from build123d import *

# Parameters (mm, degrees)
F0_W     = 62
F0_H     = 36
F1_DEPTH = 32
F2_W     = 60
F2_H     = 30
F3_DEPTH = 36.001
F5_DEPTH = 12.001
F6_W     = 16
F6_H     = 12
F7_DEPTH = 12.001
F8_R     = 8
F9_DEPTH = 12.001
F10_R    = 5


with BuildPart() as f1:
    # F0 (on Top) → F1 (new body)
    with BuildSketch(Plane.XY):
        with Locations((-13, 0)):
            Rectangle(F0_W, F0_H)
    extrude(amount=F1_DEPTH)

    # F2 (on face) → F3 (cut, through all)
    with BuildSketch(Plane.XZ.offset(18)):
        with Locations((-2, 27)):
            Rectangle(F2_W, F2_H)
    extrude(amount=-F3_DEPTH, mode=Mode.SUBTRACT)

    # F4 (on face) → F5 (cut, through all)
    with BuildSketch(Plane.XY.offset(12)):
        with BuildLine():
            ThreePointArc((0, 18), (18, 0), (0, -18))
            Line((0, -18), (0, -28))
            Line((0, -28), (28, -28))
            Line((28, -28), (28, 28))
            Line((28, 28), (0, 28))
            Line((0, 28), (0, 18))
        make_face()
    extrude(amount=-F5_DEPTH, mode=Mode.SUBTRACT)

    # F6 (on face) → F7 (cut, through all)
    with BuildSketch(Plane.YZ.offset(-32)):
        with Locations((0, 30)):
            Rectangle(F6_W, F6_H)
    extrude(amount=-F7_DEPTH, mode=Mode.SUBTRACT)

    # F8 (on face) → F9 (cut, through all)
    with BuildSketch(Plane.XY.offset(12)):
        Circle(F8_R)
    extrude(amount=-F9_DEPTH, mode=Mode.SUBTRACT)

    # F10
    f10_edges = [f1.edges().sort_by_distance(p)[0] for p in [
        (-38, 18, 32),
        (-38, -18, 32),
    ]]
    fillet(f10_edges, radius=F10_R)


solid = f1.part
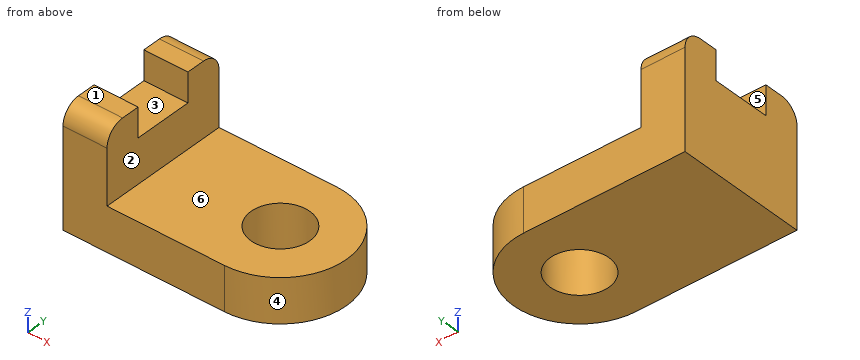
Model file for the job. Use its own axes, mm. Face numbers are marked on the shaded views. A direction names the side the tool comes from. Give positions to 0.01 mm unless a question says otherwise; leave off trailing zeros. Order: outer loops, then holes, each group sorted by start corner. A loop starts at its lowest first (then second) coordinate and runs counter-clockwise, first axis right, second up. Notation, with made-up numbers: (65, -25) - (89, -25) arc R12 ccw to (89, -14) - close; hole circle Ø1 at (-15, 53.25). An arc over 180 degrees is marked (long way). Write item = value, one per line. Start each with the question number.
1. Cut at C-C, the plane x = -37.5. List the corners of the cut face in (y, z), and give its area (3 significant figures).
2. Cut at D-D, the plane y = 6. List the corners of the cut face in (x, z).
3. Cut at B-B, the plane x = -4. List the corners of the cut face in (y, z), and give its area (3 significant figures).
4. Which spindle directions (+Z, -Z, +X, -X, +Y, -Y) get a long thin tool onto all of the face, cutting with end or side? Do the marked faces 1, 2 and 3. Say none if no direction does.
5. Probe line 1 along Y through (x, z) = (0, 6); line 2 along X through (y, z) = (-16, 30.5); line 3 along X through (y, z) = (-5, 7) (3 decimals). List the from-to ranges inside material, lowest first.
6. Cut at A-A, the plane y = 0. List the corners of the cut face in (x, z), and give its area (3 significant figures).
7. Two-plate mould, pull along Y, no slides. Class the marked faces 4, 5 and 6: pulls with the +Y half, pulls with the -Y half, needs draft (parallel to the pull), parting line crosses it, or undercut.
8. Drop flat-ended pins along their axis: P1, Ø6, axis at y = -9, z = 8.5, coming from the +X side; P2, Ø6, axis at y = -7, z = 19, coming from the +X side; P3, Ø1.5, axis at x = 3.5, y = -11, coming from the +Z side. Give the stop position or say it passes through.
Taken from the geometry:
q1.outline = (-18, 0) - (18, 0) - (18, 27) arc R5 ccw to (13, 32) - (8, 32) - (8, 24) - (-8, 24) - (-8, 32) - (-13, 32) arc R5 ccw to (-18, 27) - close
q1.area = 1,010 mm²
q2.outline = (-44, 0) - (-5.29, 0) - (-5.29, 12) - (-32, 12) - (-32, 24) - (-44, 24) - close; (5.29, 0) - (16.97, 0) - (16.97, 12) - (5.29, 12) - close
q3.outline = (-18, 0) - (-6.93, 0) - (-6.93, 12) - (-18, 12) - close; (6.93, 0) - (18, 0) - (18, 12) - (6.93, 12) - close
q3.area = 266 mm²
q4.face_1 = +Z, +X, -X, +Y, -Y
q4.face_2 = +Z, +X, +Y, -Y
q4.face_3 = +Z, +X, -X
q5.line_1 = -18 to -8, 8 to 18
q5.line_2 = -44 to -32
q5.line_3 = -44 to -6.245, 6.245 to 17.292
q6.outline = (-44, 0) - (-8, 0) - (-8, 12) - (-32, 12) - (-32, 24) - (-44, 24) - close; (8, 0) - (18, 0) - (18, 12) - (8, 12) - close
q6.area = 696 mm²
q7.face_4 = parting line crosses it
q7.face_5 = undercut
q7.face_6 = needs draft
q8.P1 = 16.97
q8.P2 = -32
q8.P3 = 12
